For this review, use the dimensioned drawing (mm, ordinates from the lowest corner) and the shaded views. A direction names the side the tool comes from. Round coordinates to 2 decimals unless told otherwise and drop trailing zeros. Order: outer loops, then holes, each group sorted by start corner. A loop starts at its lowest first (then second) coordinate and runs counter-clockwise, first axis right, second up. Notation, with made-up numbers: M 55.25,53.5 L 110.25,53.5 A25 ccw 110.25,75.5 Z; hole C 7,80.25 d4. An arc over 180 degrees is marked long. Put each result on its own line as item: value.
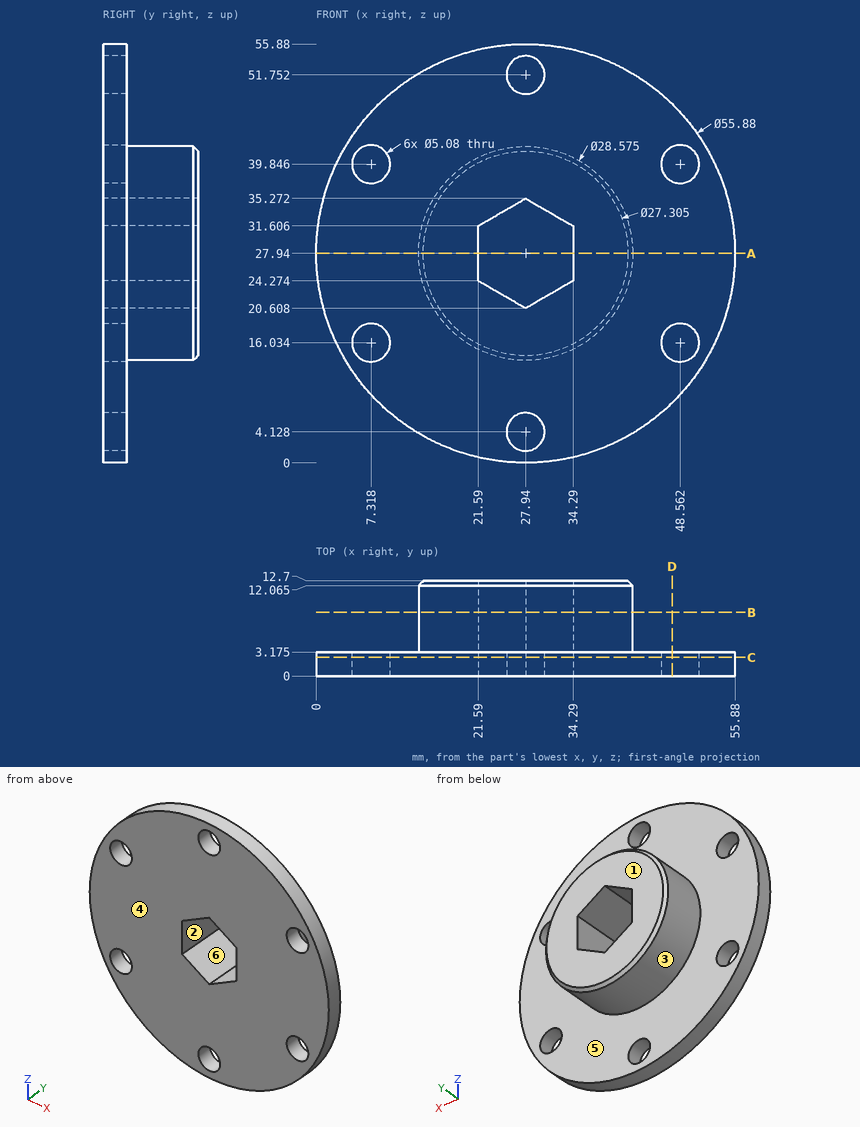
(1) Add section A-A on z = 27.94. Give the boundary of the cut face in (x, y) (1 decimal).
A:
outline: M 0,0 L 21.6,0 L 21.6,12.7 L 14.3,12.7 L 13.7,12.1 L 13.7,3.2 L 0,3.2 Z; M 34.3,0 L 55.9,0 L 55.9,3.2 L 42.2,3.2 L 42.2,12.1 L 41.6,12.7 L 34.3,12.7 Z
(2) For the marked faces 4, 5 and 6, list the 3-axis set-ups (+Z, -Z, +X, -X, +Y, -Y) from which the entire face can be reached by the end or side of a thin tool; tool diameter is ignored.
A:
face 4: +Z, -Z, +X, -X, -Y
face 5: +Y
face 6: +Y, -Y
(3) Insertion check: pin 1 Ø3 at (x, z) = (7.32, 39.85) entering from +Y; pin 2 Ø6.5 at (x, z) = (27.94, 51.75) entering from -Y; pin 3 Ø2 at (y, z) = (5.5, 26.5) entering from -X; pin 4 Ø10 at (x, z) = (39.5, 46) entering from +Y (1 decimal). Each pin has a flat end and moves straight along its axis. Give the tip position at first contact, or say it passes through.
A:
pin 1: passes through
pin 2: stops at y = 0
pin 3: stops at x = 13.66
pin 4: stops at y = 3.2
(4) Add section D-D on x = 47.5. Give the boundary of the cut face in (y, z) (1 decimal).
A:
outline: M 0,8 L 3.2,8 L 3.2,13.7 L 0,13.7 Z; M 0,18.3 L 3.2,18.3 L 3.2,37.5 L 0,37.5 Z; M 0,42.2 L 3.2,42.2 L 3.2,47.9 L 0,47.9 Z
(5) Draft analysis for pull direction Z (two halves, no side actions). For the marked faces 1, 2 and 3, state which applies: released by +Z, released by -Z, zero draft, split by the parting line, or undercut.
A:
face 1: zero draft
face 2: undercut
face 3: split by the parting line
(6) Add section B-B on y = 8.5. Give the boundary of the cut face in (x, z) (1 decimal).
A:
outline: C 27.9,27.9 d28.6; hole M 21.6,24.3 L 27.9,20.6 L 34.3,24.3 L 34.3,31.6 L 27.9,35.3 L 21.6,31.6 Z
(7) Add section C-C on y = 2.5. Give the boundary of the cut face in (x, z), then the cut area to 3 significant figures.
A:
outline: C 27.94,27.94 d55.88; hole C 7.32,16.03 d5.08; hole C 7.32,39.85 d5.08; hole M 21.59,24.27 L 27.94,20.61 L 34.29,24.27 L 34.29,31.61 L 27.94,35.27 L 21.59,31.61 Z; hole C 27.94,4.13 d5.08; hole C 27.94,51.75 d5.08; hole C 48.56,16.03 d5.08; hole C 48.56,39.85 d5.08
area: 2,190 mm2
(8) To check wall thickness, follow L1, parallel to Y at x = 47, z = 20 (1 decimal); L2, parallel to X at y = 5.5, z = 24.5; L3, parallel to Z at x = 27.5, y = 12.25 (1 decimal). State the ranges of each line that lie inside material, in increasing order.
A:
L1: y = 0 to 3.2
L2: x = 14.07 to 21.59, 34.29 to 41.81
L3: z = 13.8 to 20.9, 35 to 42
